Design review of the part built by this model. Coordinates are the model's own, in mm. Coordinates: 2 decimals unless noted, no trailing zeros. Order: outer loops, then holes, each group sorted by start corner. A loop starts at its lowest first (then second) coordinate and runs counter-clockwise, first axis right, second up. Notation, with made-up numbers: M -24.75,47.25 L -18.75,47.25 A17 ccw -18.75,55.25 Z; hole C 58,-19 d7. An arc over 180 degrees is marked long. Answer in a Markdown table with one row per item.
from build123d import *

# Parameters (mm, degrees)
SKETCH1_W                    = 54.61
SKETCH1_H                    = 54.61
BOSS_EXTRUDE1_DEPTH          = 6.35
F_10_0_1935_DIAMETER_HOLE1_D = 4.9149
F_32_0_116_DIAMETER_HOLE1_D  = 2.9464
SKETCH10_R                   = 2.5781
CUT_EXTRUDE1_DEPTH           = 6.35


with BuildPart() as part:
    # Sketch1 → Boss-Extrude1 (new body)
    with BuildSketch(Plane.XY):
        Rectangle(SKETCH1_W, SKETCH1_H)
    extrude(amount=BOSS_EXTRUDE1_DEPTH)

    # #10 (0.1935) Diameter Hole1 (through all)
    with Locations(Plane.XY.offset(6.35)):
        with Locations((-23.5458, 23.5458), (23.510742074, 23.5458), (23.510742074, -23.510742074), (-23.5458, -23.510742074)):
            Hole(F_10_0_1935_DIAMETER_HOLE1_D / 2)

    # #32 (0.116) Diameter Hole1 (through all)
    with Locations(Plane.XY.offset(6.35)):
        with Locations((-15.487883014, 15.494), (15.494, 15.487883014), (15.487883014, -15.494), (-15.494, -15.487883014)):
            Hole(F_32_0_116_DIAMETER_HOLE1_D / 2)

    # Sketch10 → Cut-Extrude1 (cut)
    with BuildSketch(Plane.XY):
        with Locations((0, 6.35)):
            Circle(SKETCH10_R)
        with Locations((0, -6.35)):
            Circle(SKETCH10_R)
    extrude(amount=CUT_EXTRUDE1_DEPTH, mode=Mode.SUBTRACT)


solid = part.part
(1) Add section D-D, the plane y = 8. Give the boundary of the cut face in (x, z) (3 decimals).
Return value:
| item | result |
|---|---|
| outline | M -27.305,0 L -1.981,0 L -1.981,6.35 L -27.305,6.35 Z; M 1.981,0 L 27.305,0 L 27.305,6.35 L 1.981,6.35 Z |
(2) Add section C-C, the plane z = 5. Give the number of separate pieces and of enclosed holes in the cut face, and give its area (3 significant figures).
Return value:
| item | result |
|---|---|
| separate pieces | 1 |
| enclosed holes | 10 |
| area | 2,840 mm2 |
(3) Draft analysis for pull direction Y (two halves, no side actions). For faces 1 (the flat face through (0, -27.305, 3)), 2 (the cylindrical face through (-0.559, 3.833, 3.131)), 3 (the flat face through (27.305, 0, 3)), state which applies: pulls with the +Y half, pulls with the -Y half, needs draft (parallel to the pull), parting line crosses it, or undercut.
Return value:
| item | result |
|---|---|
| face 1 | pulls with the -Y half |
| face 2 | undercut |
| face 3 | needs draft |
(4) Add section B-B, the plane y = -6.35. Give the boundary of the cut face in (x, z) (3 decimals).
Return value:
| item | result |
|---|---|
| outline | M -27.305,0 L -2.578,0 L -2.578,6.35 L -27.305,6.35 Z; M 2.578,0 L 27.305,0 L 27.305,6.35 L 2.578,6.35 Z |
(5) For line 1 along Y through (x, z) = (23.5, 5.5) (3 decimals); line 2 along X through (y, z) = (22, 4) (3 decimals); line 3 along Y through (x, z) = (-16, 3.25) (3 decimals), list the stretches that pass through material, from the lowest coordinate up. Write a range as from..to.
Return value:
| item | result |
|---|---|
| line 1 | y = -27.305..-25.968, -21.053..21.088, 26.003..27.305 |
| line 2 | x = -27.305..-25.456, -21.635..21.6, 25.421..27.305 |
| line 3 | y = -27.305..-16.871, -14.104..14.113, 16.875..27.305 |
(6) Add section A-A, the plane x = 0. Give the boundary of the cut face in (y, z) (3 decimals), and give its area (3 significant figures).
Return value:
| item | result |
|---|---|
| outline | M -27.305,0 L -8.928,0 L -8.928,6.35 L -27.305,6.35 Z; M -3.772,0 L 3.772,0 L 3.772,6.35 L -3.772,6.35 Z; M 8.928,0 L 27.305,0 L 27.305,6.35 L 8.928,6.35 Z |
| area | 281 mm2 |
